```python
from build123d import *

# Parameters (mm, degrees)
SKETCH1_W           = 180
SKETCH1_H           = 68.4
SKETCH1_R           = 3.302
BOSS_EXTRUDE1_DEPTH = 1
SKETCH2_R           = 11.5
SKETCH2_R_2         = 1.6
CUT_EXTRUDE1_DEPTH  = 1
LPATTERN1_COUNT     = 3
LPATTERN1_PITCH     = 69


with BuildPart() as part:
    # Sketch1 → Boss-Extrude1 (new body)
    with BuildSketch(Plane.XY):
        with Locations((90, 34.2)):
            Rectangle(SKETCH1_W, SKETCH1_H)
        with Locations((21, 12.7)):
            Circle(SKETCH1_R, mode=Mode.SUBTRACT)
        with Locations((90, 12.7)):
            Circle(SKETCH1_R, mode=Mode.SUBTRACT)
        with Locations((159, 12.7)):
            Circle(SKETCH1_R, mode=Mode.SUBTRACT)
    extrude(amount=BOSS_EXTRUDE1_DEPTH)

    # Sketch2 → Cut-Extrude1 (cut)
    with BuildSketch(Plane.XY.offset(1)):
        with Locations((21, 47.4)):
            Circle(SKETCH2_R)
        with Locations((36.5, 62.9)):
            Circle(SKETCH2_R_2)
        with Locations((36.5, 31.9)):
            Circle(SKETCH2_R_2)
        with Locations((5.5, 31.9)):
            Circle(SKETCH2_R_2)
        with Locations((5.5, 62.9)):
            Circle(SKETCH2_R_2)
    cut_extrude1 = extrude(amount=-CUT_EXTRUDE1_DEPTH, mode=Mode.SUBTRACT)

    # LPattern1: Cut-Extrude1 ×3
    with Locations(*[(i * LPATTERN1_PITCH, 0, 0) for i in range(1, LPATTERN1_COUNT)]):
        add(cut_extrude1, mode=Mode.SUBTRACT)


solid = part.part
```
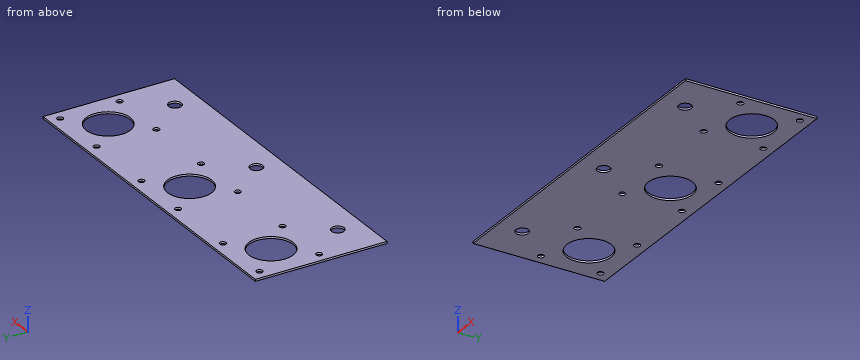
The listing builds one solid part. Answer for the finished solid, in the listing's coordinates (mm). Round coordinates to 2 decimals unless told otherwise and drop trailing zeros. Write each loop counter-clockwise with the first axis right and the second up, starting at its lowest first coordinate (ties: lowest second). Pieces come first, ordered by that corner, then holes. Notation, with made-up numbers: (-16.5, -13) -> (-1.5, -13) arc R28 ccw to (-1.5, 14) -> close; hole circle Ø9 at (15.25, 85.25). An arc over 180 degrees is marked (long way). Answer as a JSON object with one key per item and string values. Group by question number.
Q1. Section D-D (y = 47.4) is taken. Write down the section's boundary in (x, z), plus the area to 3 significant figures.
Q2. Straight lines are drawn through the part: line 1 along Y through (x, z) = (21, 0.45); line 2 along Y through (x, z) = (36.5, 0.7); line 3 along X through (y, z) = (42, 0.2). For each, find the intervals that lie inside material, in ascending order.
Q3. This flat-tipped pin is pushed along its axis until it touches: pin 1 Ø1.9 at (x, y) = (143.5, 31.9) entering from +Z. Where does it stop, or does it pass through?
Q4. Section A-A (y = 12.7) is taken. Write down the section's boundary in (x, z), plus the area to 3 significant figures.
Q5. Section C-C (x = 5.5) is taken. Write down the section's boundary in (y, z), plus the area to 3 significant figures.
Q6. Section B-B (z = 0.65) is taken. Count the separate pieces of the cut face and the enclosed holes in it, plus the area to 3 significant figures.
Check values:
{
 "1": {"outline": "(0, 0) -> (9.5, 0) -> (9.5, 1) -> (0, 1) -> close; (32.5, 0) -> (78.5, 0) -> (78.5, 1) -> (32.5, 1) -> close; (101.5, 0) -> (147.5, 0) -> (147.5, 1) -> (101.5, 1) -> close; (170.5, 0) -> (180, 0) -> (180, 1) -> (170.5, 1) -> close", "area": "111 mm^2"},
 "2": {"line 1": "0 to 9.4, 16 to 35.9, 58.9 to 68.4", "line 2": "0 to 30.3, 33.5 to 61.3, 64.5 to 68.4", "line 3": "0 to 10.85, 31.15 to 79.85, 100.15 to 148.85, 169.15 to 180"},
 "3": {"pin 1": "through"},
 "4": {"outline": "(0, 0) -> (17.7, 0) -> (17.7, 1) -> (0, 1) -> close; (24.3, 0) -> (86.7, 0) -> (86.7, 1) -> (24.3, 1) -> close; (93.3, 0) -> (155.7, 0) -> (155.7, 1) -> (93.3, 1) -> close; (162.3, 0) -> (180, 0) -> (180, 1) -> (162.3, 1) -> close", "area": "160 mm^2"},
 "5": {"outline": "(0, 0) -> (30.3, 0) -> (30.3, 1) -> (0, 1) -> close; (33.5, 0) -> (61.3, 0) -> (61.3, 1) -> (33.5, 1) -> close; (64.5, 0) -> (68.4, 0) -> (68.4, 1) -> (64.5, 1) -> close", "area": "62.0 mm^2"},
 "6": {"separate pieces": "1", "enclosed holes": "18", "area": "10,900 mm^2"}
}
